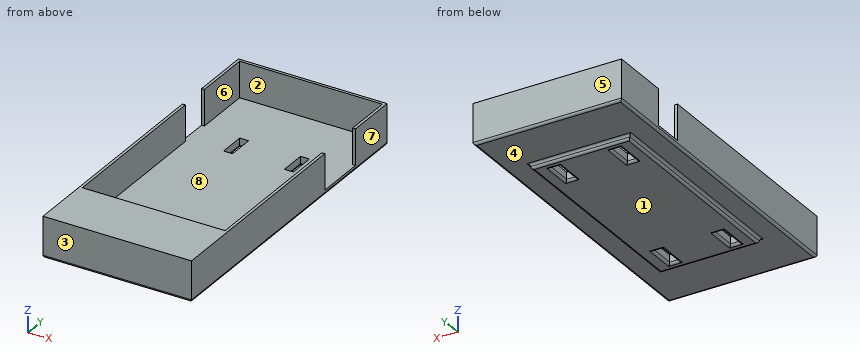
```python
from build123d import *

# Parameters (mm, degrees)
F0_W     = 62.1875934303
F0_H     = 133.9231580496
F1_DEPTH = 2
F3_DEPTH = 15
F4_W     = 62.1875934303
F4_H     = 1.7857002169
F5_DEPTH = 25
F6_W     = 41.5440425277
F6_H     = 88.6942744255
F7_DEPTH = 2
F8_W     = 3.7540234625
F8_H     = 11.0563002527
F9_DEPTH = 8
F10_R    = 0.99999


# Not quite as in the source:
# - a fillet or chamfer is up to 0.001 mm smaller than in the source, because OpenCascade refuses the exact size


with BuildPart() as f1:
    # F0 (on Top) → F1 (new body)
    with BuildSketch(Plane.XY):
        Rectangle(F0_W, F0_H)
    extrude(amount=F1_DEPTH)

    # F2 (on face) → F3 (join)
    with BuildSketch(Plane.XY.offset(2)):
        Polygon((29.8937967151, 45.4372726381), (31.0937967151, 45.4372726381), (31.0937967151, 66.9615790248), (-31.0937967151, 66.9615790248), (-31.0937967151, 41.7135171592), (-29.8937967151, 41.7135171592), (-29.8937967151, 65.7615790248), (29.8937967151, 65.7615790248), align=None)
        Polygon((-31.0937967151, -66.9615790248), (31.0937967151, -66.9615790248), (31.0937967151, 24.3710856885), (29.8937967151, 24.3710856885), (29.8937967151, -65.7615790248), (-29.8937967151, -65.7615790248), (-29.8937967151, 28.5614430904), (-31.0937967151, 28.5614430904), align=None)
    extrude(amount=F3_DEPTH)

    # F4 (on face) → F5 (join)
    with BuildSketch(Plane.XZ.offset(66.9615790248)):
        with Locations((0, 16.1071498916)):
            Rectangle(F4_W, F4_H)
    extrude(amount=-F5_DEPTH)

    # F6 (on face) → F7 (join)
    with BuildSketch(Plane(origin=(0, 0, 0), x_dir=(1, 0, 0), z_dir=(0, 0, -1))):
        Rectangle(F6_W, F6_H)
    extrude(amount=F7_DEPTH)

    # F8 (on face) → F9 (cut)
    with BuildSketch(Plane(origin=(0, 0, -2), x_dir=(1, 0, 0), z_dir=(0, 0, -1))):
        with Locations((12.7368234098, -35.2913737297)):
            Rectangle(F8_W, F8_H)
        with Locations((-12.7368234098, -35.2913737297)):
            Rectangle(F8_W, F8_H)
        with Locations((-12.7368234098, 35.2913737297)):
            Rectangle(F8_W, F8_H)
        with Locations((12.7368234098, 35.2913737297)):
            Rectangle(F8_W, F8_H)
    extrude(amount=-F9_DEPTH, mode=Mode.SUBTRACT)

    # F10 (radius 1 in the source; OpenCascade refuses exactly that, so slightly less here)
    f10_edges = [f1.edges().sort_by_distance(p)[0] for p in [
        (0, -44.347137, -2),
        (20.772021, 0, -2),
        (-20.772021, 0, -2),
        (0, 44.347137, -2),
        (-10.859812, 35.291374, -2),
        (-12.736823, 29.763224, -2),
        (-14.613835, 35.291374, -2),
        (-12.736823, 40.819524, -2),
        (12.736823, 29.763224, -2),
        (10.859812, 35.291374, -2),
        (12.736823, 40.819524, -2),
        (14.613835, 35.291374, -2),
        (-12.736823, -29.763224, -2),
        (-10.859812, -35.291374, -2),
        (-12.736823, -40.819524, -2),
        (-14.613835, -35.291374, -2),
        (12.736823, -29.763224, -2),
        (14.613835, -35.291374, -2),
        (12.736823, -40.819524, -2),
        (10.859812, -35.291374, -2),
        (-31.093797, 0, 0),
        (0, 66.961579, 0),
        (0, -66.961579, 0),
        (31.093797, 0, 0),
        (20.772021, 0, 0),
        (0, 44.347137, 0),
        (-20.772021, 0, 0),
        (0, -44.347137, 0),
    ]]
    fillet(f10_edges, radius=F10_R)


solid = f1.part
```
Work out the finished part from the listing and answer in its coordinate system (mm). Face numbers are marked on the shaded views. A direction names the side the tool comes from. Coordinates: 2 decimals unless noted, no trailing zeros. Loops run counter-clockwise (first coordinate to the right, second up) from the corner with the lowest first, then second, coordinate; pieces in that order, holes last. Notation, with made-up numbers: (5, 45.25) -> (37, 45.25) arc R25 cw to (37, 65.25) -> close; hole circle Ø4 at (32.25, 41). An arc over 180 degrees is marked (long way). Answer as CSV lines item,"result".
Q1. The part is cut by section B-B on z = 14. Write down the section's boundary in (x, y).
Findings:
outline,"(-31.09, -66.96) -> (31.09, -66.96) -> (31.09, 24.37) -> (29.89, 24.37) -> (29.89, -65.76) -> (-29.89, -65.76) -> (-29.89, 28.56) -> (-31.09, 28.56) -> close; (-31.09, 41.71) -> (-29.89, 41.71) -> (-29.89, 65.76) -> (29.89, 65.76) -> (29.89, 45.44) -> (31.09, 45.44) -> (31.09, 66.96) -> (-31.09, 66.96) -> close"
Q2. Find the intervals of material crossed by probe 1 along Y at (x, z) = (-21, 11); probe 2 along Y at (x, z) = (8, 15.75); probe 3 along X at (y, z) = (22, 7.5), in increasing order.
Findings:
probe 1,"y = -66.96 to -65.76, 65.76 to 66.96"
probe 2,"y = -66.96 to -41.96, 65.76 to 66.96"
probe 3,"x = -31.09 to -29.89, 29.89 to 31.09"
Q3. For a pull along Y with two mould halves and no side action, classify the marked faces 1, 2 and 3 as +Y half, -Y half, draft (parallel to the pull), parting line (faces both ways), or undercut.
Findings:
face 1,"draft"
face 2,"undercut"
face 3,"-Y half"
Q4. Each of these flat-tipped pins is pushed along its axis until it touches: pin 1 (4 mm diameter, centred on y = 25.5, z = 5, fed in from +X); pin 2 (12 mm diameter, centred on x = -1, y = 51, fed in from +Z). Where does it stop, or does it pass through?
Findings:
pin 1,"stops at x = 31.09"
pin 2,"stops at z = 2"
Q5. A tool of negligible diameter and unlimited length cuts with its end or side. For the marked faces 4, 5, 6, 7 and 8, from which of +Z, -Z, +X, -X, +Y, -Y can it reach the whole face along a straight path? Write none if from no direction.
Findings:
face 4,"-Z"
face 5,"+Z, -Z, +X, -X, +Y"
face 6,"+Z"
face 7,"+Z, -Z, +X, +Y, -Y"
face 8,"none"
Q6. The part is cut by section A-A on y = -39. State how many separate pieces and enclosed holes the cut face has, and give its area (3 significant figures).
Findings:
separate pieces,"3"
enclosed holes,"0"
area,"212 mm²"
